The figure shows three views and two pictorial views of one solid part (mm, origin at its lowest corner). Answer the questions. A direction names the side the tool comes from. Round coordinates to 2 decimals unless told otherwise and drop trailing zeros. Loops run counter-clockwise (first coordinate to the right, second up) from the corner with the lowest first, then second, coordinate; pieces in that order, holes last. Notation, with made-up numbers: (5, 8.5) -> (53, 8.5) arc R38 ccw to (53, 47.5) -> close; hole circle Ø8 at (37.25, 15). An arc over 180 degrees is marked (long way). Write item = value, one per line. Start each with the question number.
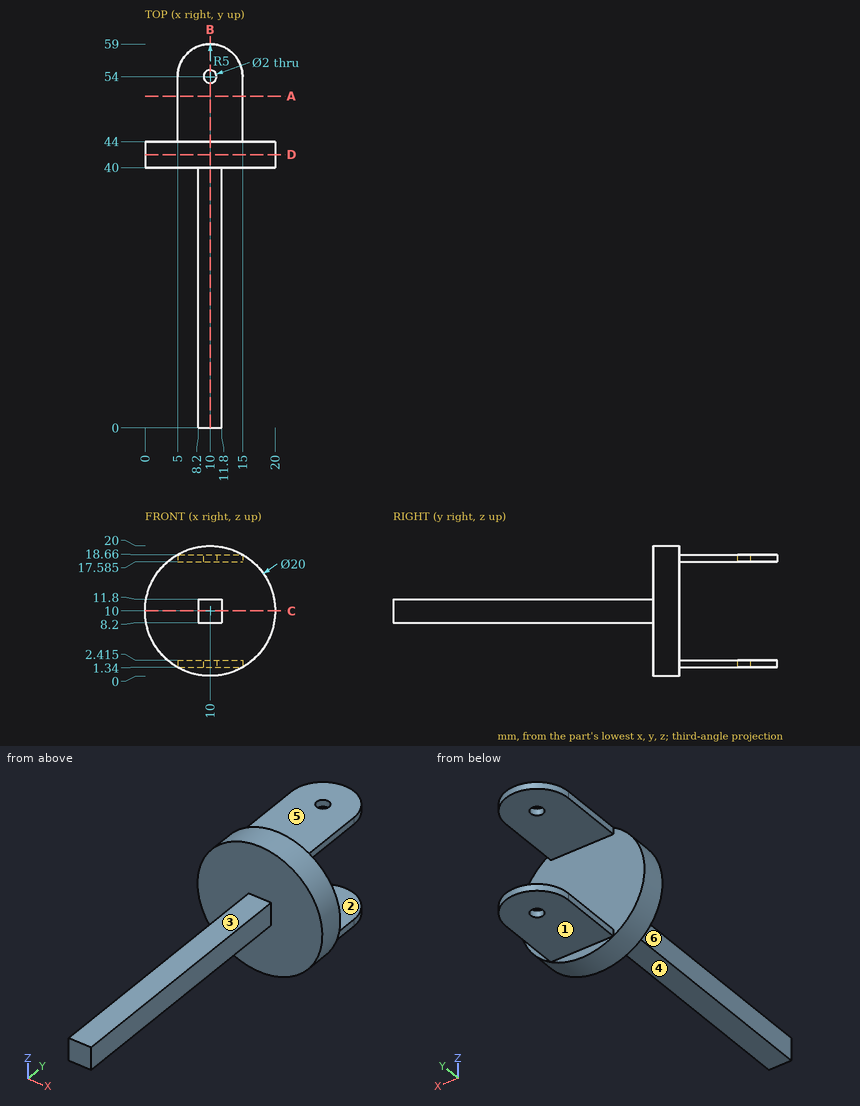
Item 1: Flat-ended cylindrical pins translate along their axes: pin 1 (6 mm diameter, centred on x = 14, y = 50, fed in from +Z); pin 2 (5 mm diameter, centred on x = 9, y = 50, fed in from -Z); pin 3 (3 mm diameter, centred on x = 15.5, z = 17.5, fed in from +Y). Find the tip coordinate at first contact, or state that the pin passes through.
Item 2: The mould has two halves that part along Z. Classify the marked faces 1, 2 and 3: pulls with the +Z half, pulls with the -Z half, needs draft (parallel to the pull), parting line crosses it, or undercut.
Item 3: Section D-D (y = 42) is taken. Determine the outline of the cut face in (x, z), then the cut area to 3 significant figures.
Item 4: Section C-C (z = 10) is taken. Determine the outline of the cut face in (x, y).
Item 5: Find the intervals of material crossed by line 1 along Y through (x, z) = (10, 18.05); line 2 along Y through (x, z) = (16.5, 17); line 3 along Z through (x, y) = (9, 29.5), in increasing order. Write a range as [from, to].
Item 6: Section B-B (x = 10) is taken. Determine the outline of the cut face in (y, z) (1 decimal).
Item 7: A tool of negligible diameter and unlimited length cuts with its end or side. For the marked faces 4, 5 and 6, from which of +Z, -Z, +X, -X, +Y, -Y can it reach the whole face along a straight path? Write none if from no direction.
Item 8: Section A-A (y = 51) is taken. Determine the outline of the cut face in (x, z) (1 decimal), then the cut area to 3 significant figures.
Worked answers:
q1.pin_1 = 18.66
q1.pin_2 = 1.34
q1.pin_3 = 57
q2.face_1 = pulls with the -Z half
q2.face_2 = undercut
q2.face_3 = pulls with the +Z half
q3.outline = circle Ø20 at (10, 10)
q3.area = 314 mm2
q4.outline = (0, 40) -> (8.2, 40) -> (8.2, 0) -> (11.8, 0) -> (11.8, 40) -> (20, 40) -> (20, 44) -> (0, 44) -> close
q5.line_1 = [40, 53], [55, 59]
q5.line_2 = [40, 44]
q5.line_3 = [8.2, 11.8]
q6.outline = (0, 8.2) -> (40, 8.2) -> (40, 0) -> (44, 0) -> (44, 1.3) -> (53, 1.3) -> (53, 2.4) -> (44, 2.4) -> (44, 17.6) -> (53, 17.6) -> (53, 18.7) -> (44, 18.7) -> (44, 20) -> (40, 20) -> (40, 11.8) -> (0, 11.8) -> close; (55, 1.3) -> (59, 1.3) -> (59, 2.4) -> (55, 2.4) -> close; (55, 17.6) -> (59, 17.6) -> (59, 18.7) -> (55, 18.7) -> close
q7.face_4 = -Z, +X, -X, -Y
q7.face_5 = +Z, +X, -X, +Y
q7.face_6 = +Z, -Z, -X, -Y
q8.outline = (5, 1.3) -> (15, 1.3) -> (15, 2.4) -> (5, 2.4) -> close; (5, 17.6) -> (15, 17.6) -> (15, 18.7) -> (5, 18.7) -> close
q8.area = 21.5 mm2
